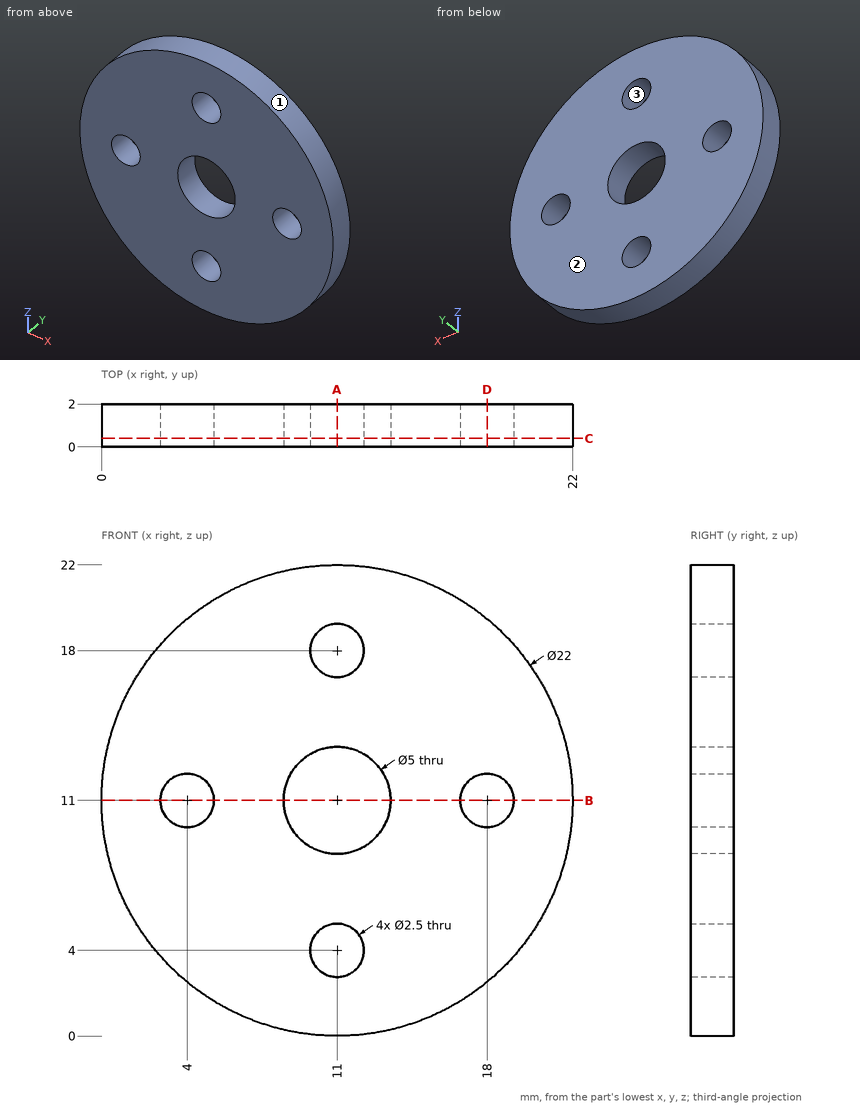
Study the drawing (mm; zero at the part's minimum x, y, z) and answer. Give positions to 0.01 mm unless a question says otherwise; leave off trailing zeros. Order: outer loops, then holes, each group sorted by start corner. A loop starts at its lowest first (then second) coordinate and runs counter-clockwise, first axis right, second up. Notation, with made-up numbers: (78, 67.25) - (124, 67.25) arc R26 cw to (124, 99.25) - close; hole circle Ø9 at (-2, -37). An arc over 180 degrees is marked (long way). Answer in a Markdown table with one row per item. Add a question column.
Q1. Find the intervals of material crossed by line 1 along X through (y, z) = (1.45, 11); line 2 along X through (y, z) = (1.55, 10); line 3 along Z through (x, y) = (10.5, 1.75), in increasing order. Write a range as [from, to].
Q2. For a pull along X with two mould halves and no side action, classify the marked faces 1, 2 and 3 as released by +X, released by -X, zero draft, split by the parting line, or undercut.
Q3. The part is cut by section C-C (y = 0.4). Determine the outline of the cut face in (x, z), then the cut area to 3 significant figures.
Q4. The part is cut by section D-D (x = 18). Determine the outline of the cut face in (y, z), then the cut area to 3 significant figures.
Q5. The part is cut by section A-A (x = 11). Determine the outline of the cut face in (y, z).
Q6. The part is cut by section B-B (z = 11). Determine the outline of the cut face in (x, y).
Determined:
| question | item | result |
|---|---|---|
| 1 | line 1 | x = [0, 2.75], [5.25, 8.5], [13.5, 16.75], [19.25, 22] |
| 1 | line 2 | x = [0.05, 3.25], [4.75, 8.71], [13.29, 17.25], [18.75, 21.95] |
| 1 | line 3 | z = [0.01, 2.85], [5.15, 8.55], [13.45, 16.85], [19.15, 21.99] |
| 2 | face 1 | split by the parting line |
| 2 | face 2 | zero draft |
| 2 | face 3 | undercut |
| 3 | outline | circle Ø22 at (11, 11); hole circle Ø2.5 at (4, 11); hole circle Ø5 at (11, 11); hole circle Ø2.5 at (11, 4); hole circle Ø2.5 at (11, 18); hole circle Ø2.5 at (18, 11) |
| 3 | area | 341 mm² |
| 4 | outline | (0, 2.51) - (2, 2.51) - (2, 9.75) - (0, 9.75) - close; (0, 12.25) - (2, 12.25) - (2, 19.49) - (0, 19.49) - close |
| 4 | area | 28.9 mm² |
| 5 | outline | (0, 0) - (2, 0) - (2, 2.75) - (0, 2.75) - close; (0, 5.25) - (2, 5.25) - (2, 8.5) - (0, 8.5) - close; (0, 13.5) - (2, 13.5) - (2, 16.75) - (0, 16.75) - close; (0, 19.25) - (2, 19.25) - (2, 22) - (0, 22) - close |
| 6 | outline | (0, 0) - (2.75, 0) - (2.75, 2) - (0, 2) - close; (5.25, 0) - (8.5, 0) - (8.5, 2) - (5.25, 2) - close; (13.5, 0) - (16.75, 0) - (16.75, 2) - (13.5, 2) - close; (19.25, 0) - (22, 0) - (22, 2) - (19.25, 2) - close |
